from build123d import *

# Parameters (mm, degrees)
F0_W     = 160
F0_H     = 150
F1_DEPTH = 8
F3_R     = 2
F4_DEPTH = 8.001


with BuildPart() as f1:
    # F0 (on Top) → F1 (new body)
    with BuildSketch(Plane.XY):
        with Locations((70.181546, 27.561349)):
            Rectangle(F0_W, F0_H)
    extrude(amount=F1_DEPTH)

    # F3 (on face) → F4 (cut, through all)
    with BuildSketch(Plane.XY.offset(8)):
        with Locations((0.181546, 92.561349)):
            Circle(F3_R)
        with Locations((40.181546, 92.561349)):
            Circle(F3_R)
        with Locations((100.181546, 92.561349)):
            Circle(F3_R)
        with Locations((140.181546, 92.561349)):
            Circle(F3_R)
        with Locations((140.181546, 52.561349)):
            Circle(F3_R)
        with Locations((100.181546, 52.561349)):
            Circle(F3_R)
        with Locations((40.181546, 52.561349)):
            Circle(F3_R)
        with Locations((0.181546, 52.561349)):
            Circle(F3_R)
        with Locations((0.181546, 2.561349)):
            Circle(F3_R)
        with Locations((40.181546, 2.561349)):
            Circle(F3_R)
        with Locations((100.181546, 2.561349)):
            Circle(F3_R)
        with Locations((140.181546, 2.561349)):
            Circle(F3_R)
        with Locations((140.181546, -37.438651)):
            Circle(F3_R)
        with Locations((100.181546, -37.438651)):
            Circle(F3_R)
        with Locations((40.181546, -37.438651)):
            Circle(F3_R)
        with Locations((0.181546, -37.438651)):
            Circle(F3_R)
    extrude(amount=-F4_DEPTH, mode=Mode.SUBTRACT)


solid = f1.part
Read the model definition and answer for the solid it produces. Units are mm, in the model's axes. Round coordinates to 2 decimals unless told otherwise and drop trailing zeros. Use a Markdown table: item, result.
(1) The mould has two halves that part along X. Classify faces 1 (the cylindrical face through (142.03, 1.8, 4.06)), 2 (the cylindrical face through (102.03, 51.8, 4.06)), 3 (the flat face through (69, 29, 8)), 4 (the flat face through (150.182, 27, 4)): released by +X, released by -X, zero draft, split by the parting line, or undercut.
Reported:
| item | result |
|---|---|
| face 1 | undercut |
| face 2 | undercut |
| face 3 | zero draft |
| face 4 | released by +X |
(2) This flat-tipped pin is pushed along its axis until it touches: pin 1 Ø3.5 at (x, y) = (100.18, 52.56) entering from -Z. Where does it stop, or does it pass through?
Reported:
| item | result |
|---|---|
| pin 1 | through |
(3) A straight line is drawn through the part: line 1 along Y through (x, z) = (98.5, 4.75). Find the intervals that lie inside material, in ascending order. Write a range as [from, to].
Reported:
| item | result |
|---|---|
| line 1 | [-47.44, -38.52], [-36.36, 1.48], [3.64, 51.48], [53.64, 91.48], [93.64, 102.56] |
